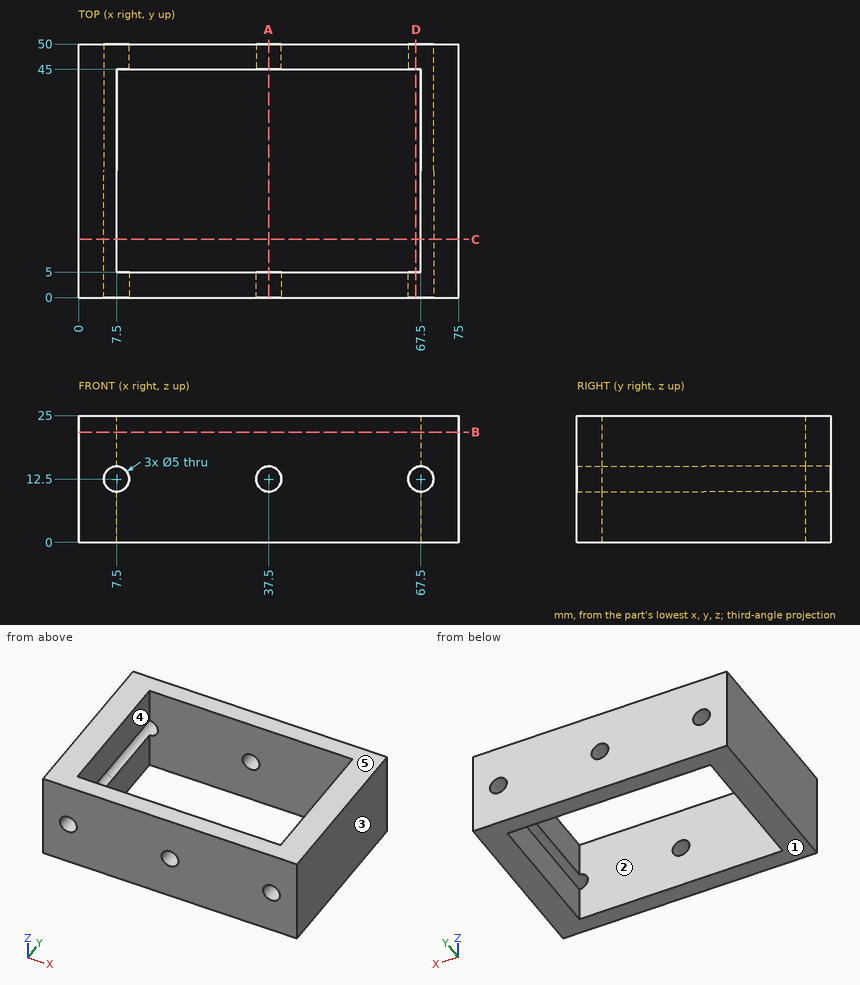
Answer from the drawing. Dimensions are ordinates in mm from the lowest x, y and z of the part. A direction names the side the tool comes from. Coordinates: 2 decimals unless noted, no trailing zeros. Write each loop counter-clockwise with the first axis right and the second up, starting at its lowest first coordinate (ties: lowest second). Pieces come first, ordered by that corner, then holes. Notation, with made-up numbers: M 2,38 L 40,38 A30 ccw 40,77 Z; hole C -39,63.25 d11. An arc over 180 degrees is marked long. Put each result on its own line as item: value. Start each with the question number.
1. A cutting plane is placed at C-C on y = 11.5. Write down the section's boundary in (x, z).
2. For a pull along X with two mould halves and no side action, classify the marked faces 3, 4 and 5 as pulls with the +X half, pulls with the -X half, needs draft (parallel to the pull), parting line crosses it, or undercut.
3. A cutting plane is placed at B-B on z = 21.75. Write down the section's boundary in (x, y), then the cut area to 3 significant figures.
4. A flat-ended cylindrical pin translates along its axis: P1, Ø4, axis at x = 32, z = 13.5, coming from the -Y side. Find the tip coordinate at first contact, or state that the pin passes through.
5. A cutting plane is placed at A-A on x = 37.5. Write down the section's boundary in (y, z), then the cut area to 3 significant figures.
6. Consider line 1 (Y direction, x = 49, z = 22.5); line 2 (X direction, y = 16.5, z = 8.25); line 3 (X direction, y = 15.5, z = 12.5). Determine where each line is inside the solid, lowest interval first. Write a range as from..to.
7. A cutting plane is placed at D-D on x = 66.5. Write down the section's boundary in (y, z).
8. Which of the six approach directions +Z, -Z, +X, -X, +Y, -Y give full straight-line access (tool end or side, diameter ignored) to the marked faces 1 and 2?
Resolved:
1. outline: M 0,0 L 7.5,0 L 7.5,10 A2.5 cw 7.5,15 L 7.5,25 L 0,25 Z; M 67.5,0 L 75,0 L 75,25 L 67.5,25 L 67.5,15 A2.5 cw 67.5,10 Z
2. face 3: pulls with the +X half
2. face 4: undercut
2. face 5: needs draft
3. outline: M 0,0 L 75,0 L 75,50 L 0,50 Z; hole M 7.5,5 L 67.5,5 L 67.5,45 L 7.5,45 Z
3. area: 1,350 mm2
4. P1: stops at y = 0
5. outline: M 0,0 L 5,0 L 5,10 L 0,10 Z; M 0,15 L 5,15 L 5,25 L 0,25 Z; M 45,0 L 50,0 L 50,10 L 45,10 Z; M 45,15 L 50,15 L 50,25 L 45,25 Z
5. area: 200 mm2
6. line 1: y = 0..5, 45..50
6. line 2: x = 0..7.5, 67.5..75
6. line 3: x = 0..5, 70..75
7. outline: M 0,0 L 5,0 L 5,10.21 L 0,10.21 Z; M 0,14.79 L 5,14.79 L 5,25 L 0,25 Z; M 45,0 L 50,0 L 50,10.21 L 45,10.21 Z; M 45,14.79 L 50,14.79 L 50,25 L 45,25 Z
8. face 1: -Z, +X, -X, +Y, -Y
8. face 2: +Z, -Z
